Part model, mm, in its own coordinate system. A direction names the side the tool comes from. Coordinates: 2 decimals unless noted, no trailing zeros. Write each loop counter-clockwise with the first axis right and the second up, starting at its lowest first coordinate (ties: lowest second). Pieces come first, ordered by that corner, then holes. Notation, with made-up numbers: (-29, -36.75) - (-25, -36.75) arc R35 cw to (-25, 0.25) - close; hole circle Ø9 at (59, -17). An arc over 180 degrees is marked (long way). Use a Markdown table: item, result.
```python
from build123d import *

# Parameters (mm, degrees)
F1_DEPTH  = 6.35
F2_R      = 10.3505
F3_DEPTH  = 3.81
F4_W      = 20.32
F4_H      = 20.066
F5_DEPTH  = 5.08
F7_DEPTH  = 12.7
F9_DEPTH  = 2.54
F10_W     = 38.1
F10_H     = 0.127
F11_DEPTH = 0.127


with BuildPart() as f1:
    # F0 (on Top) → F1 (new body)
    with BuildSketch(Plane.XY):
        Polygon((8.4455, 45.466), (-13.5255, 19.281982), (-13.5255, -30.226), (13.5255, -30.226), (13.5255, 45.466), align=None)
    extrude(amount=F1_DEPTH)

    # F2 (on face) → F3 (cut)
    with BuildSketch(Plane.XY.offset(6.35)):
        with Locations((0, -16.7005)):
            Circle(F2_R)
    extrude(amount=-F3_DEPTH, mode=Mode.SUBTRACT)

    # F4 (on face) → F5 (cut)
    with BuildSketch(Plane.XY.offset(6.35)):
        with Locations((3.3655, 10.033)):
            Rectangle(F4_W, F4_H)
    extrude(amount=-F5_DEPTH, mode=Mode.SUBTRACT)

    # F6 (on face) → F7 (cut)
    with BuildSketch(Plane(origin=(0, 45.466, 0), x_dir=(-1, 0, 0), z_dir=(0, 1, 0))):
        with BuildLine():
            ThreePointArc((-12.6365, 3.81), (-10.9855, 2.159), (-9.3345, 3.81))
            ThreePointArc((-9.3345, 3.81), (-10.9855, 5.461), (-12.6365, 3.81))
        make_face()
        with BuildLine():
            ThreePointArc((-12.6365, 3.81), (-10.9855, 5.461), (-9.3345, 3.81))
            Line((-9.3345, 3.81), (-9.3345, 6.35))
            Line((-9.3345, 6.35), (-12.6365, 6.35))
            Line((-12.6365, 6.35), (-12.6365, 3.81))
        make_face()
    extrude(amount=-F7_DEPTH, mode=Mode.SUBTRACT)

    # F8 (on face) → F9 (cut)
    with BuildSketch(Plane.XY.offset(6.35)):
        with BuildLine():
            Line((12.6365, 28.956), (12.6365, 32.766))
            Line((12.6365, 32.766), (0.441522, 32.766))
            Line((0.441522, 32.766), (-9.0805, 21.418096))
            Line((-9.0805, 21.418096), (-9.0805, -11.732868))
            ThreePointArc((-9.0805, -11.732868), (-8.063565, -10.211142), (-6.7945, -8.892324))
            Line((-6.7945, -8.892324), (-6.7945, 0))
            Line((-6.7945, 0), (-6.7945, 20.066))
            Line((-6.7945, 20.066), (0.665096, 28.956))
            Line((0.665096, 28.956), (12.6365, 28.956))
        make_face()
    extrude(amount=-F9_DEPTH, mode=Mode.SUBTRACT)

    # F10 (on face) → F11 (join)
    with BuildSketch(Plane.XY):
        with Locations((-32.5755, -30.1625)):
            Rectangle(F10_W, F10_H)
    extrude(amount=F11_DEPTH)


solid = f1.part
```
Item 1: Band-saw the part on A-A, the plane z = 5.5. Give the cut face in (x, y), then the cut area to 3 significant figures.
From the geometry:
| item | result |
|---|---|
| outline | (-13.53, -30.23) - (13.53, -30.23) - (13.53, 0) - (-6.79, 0) - (-6.79, -8.89) arc R10.35 cw (long way) to (-9.08, -11.73) - (-9.08, 21.42) - (0.44, 32.77) - (9.33, 32.77) - (9.33, 45.47) - (8.45, 45.47) - (-13.53, 19.28) - close; (-6.79, 20.07) - (13.53, 20.07) - (13.53, 45.47) - (12.64, 45.47) - (12.64, 28.96) - (0.67, 28.96) - close |
| area | 822 mm^2 |
Item 2: Band-saw the part on C-C, the plane x = -32. Give the cut face in (y, z).
From the geometry:
| item | result |
|---|---|
| outline | (-30.23, 0) - (-30.1, 0) - (-30.1, 0.13) - (-30.23, 0.13) - close |
Item 3: Drop flat-ended pins along their axis: P1, Ø2, axis at y = -6, z = 4.5, coming from the -X side; P2, Ø2, axis at y = 39, z = 5.5, coming from the -X side; P3, Ø1.3, axis at y = 13.5, z = 3, coming from the +X side. Give the stop position or say it passes through.
From the geometry:
| item | result |
|---|---|
| P1 | x = -13.53 |
| P2 | x = 2.18 |
| P3 | x = -6.79 |
Item 4: Drill centre lines: probe 1 along Y at (x, z) = (0, 4.4); probe 2 along Z at (x, y) = (-4.5, 11.5); probe 3 along Z at (x, y) = (7.5, 30). Where is each one in solid material? Low to high.
From the geometry:
| item | result |
|---|---|
| probe 1 | -30.23 to -27.05, -6.35 to 0, 20.07 to 28.16, 32.24 to 35.4 |
| probe 2 | 0 to 1.27 |
| probe 3 | 0 to 3.81 |
Item 5: Band-saw the part on B-B, the plane y = 12.5. Give the cut face in (x, z), then the cut area to 3 significant figures.
From the geometry:
| item | result |
|---|---|
| outline | (-13.53, 0) - (13.53, 0) - (13.53, 1.27) - (-6.79, 1.27) - (-6.79, 3.81) - (-9.08, 3.81) - (-9.08, 6.35) - (-13.53, 6.35) - close |
| area | 62.7 mm^2 |
Item 6: Band-saw the part on D-D, the plane y = -20.5. Give the cut face in (x, z), then the cut area to 3 significant figures.
From the geometry:
| item | result |
|---|---|
| outline | (-13.53, 0) - (13.53, 0) - (13.53, 6.35) - (9.63, 6.35) - (9.63, 2.54) - (-9.63, 2.54) - (-9.63, 6.35) - (-13.53, 6.35) - close |
| area | 98.4 mm^2 |
Item 7: Two-plate mould, pull along Y, no slides. Class faces 1 (the face through (-9.08, 5, 5)), 2 (the face through (-5, -30.226, 3)), 3 (the face through (12.636, 37, 5)): pulls with the +Y half, pulls with the -Y half, needs draft (parallel to the pull), parting line crosses it, or undercut.
From the geometry:
| item | result |
|---|---|
| face 1 | undercut |
| face 2 | pulls with the -Y half |
| face 3 | needs draft |
Item 8: Which spindle directions (+Z, -Z, +X, -X, +Y, -Y) get a long thin tool onto all of the face, cutting with end or side? Do faces 4 (the face through (9.334, 39, 5)), 5 (the face through (9.561, -20.665, 4.472)), 6 (the face through (3, 20.066, 4)). Say none if no direction does.
From the geometry:
| item | result |
|---|---|
| face 4 | +Z, +Y |
| face 5 | +Z |
| face 6 | +Z, +X |
